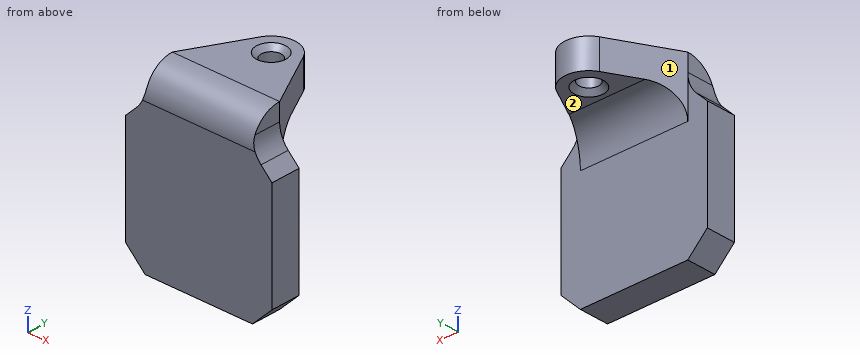
```python
from build123d import *

# Parameters (mm, degrees)
SKETCH_1_W      = 30
SKETCH_1_H      = 30
EXTRUDE_1_DEPTH = 6
CHAMFER_1_SIZE  = 4
SKETCH_2_R      = 2
EXTRUDE_2_DEPTH = 6
FILLET_1_R      = 6
FILLET_2_R      = 6
FILLET_3_R      = 6
CHAMFER_2_SIZE  = 1


with BuildPart() as part:
    # 草图1 → 凸台-拉伸1 (new body)
    with BuildSketch(Plane(origin=(0, 0, 0), x_dir=(1, 0, 0), z_dir=(0, 1, 0))):
        Rectangle(SKETCH_1_W, SKETCH_1_H)
    extrude(amount=EXTRUDE_1_DEPTH)

    # 倒角1
    chamfer_1_edges = [part.edges().sort_by_distance(p)[0] for p in [
        (15, 3, 15),
        (-15, 3, 15),
        (-15, 3, -15),
        (15, 3, -15),
    ]]
    chamfer(chamfer_1_edges, length=CHAMFER_1_SIZE)

    # 草图2 → 凸台-拉伸2 (add)
    with BuildSketch(Plane.XY.offset(15)):
        with BuildLine():
            Line((-11, 6), (-4.411764706, 18.352941176))
            ThreePointArc((-4.411764706, 18.352941176), (0, 21), (4.411764706, 18.352941176))
            Line((4.411764706, 18.352941176), (11, 6))
            Line((11, 6), (11, 0))
            Line((11, 0), (-11, 0))
            Line((-11, 0), (-11, 6))
        make_face()
        with Locations((0, 16)):
            Circle(SKETCH_2_R, mode=Mode.SUBTRACT)
    extrude(amount=EXTRUDE_2_DEPTH)

    # 圆角1
    fillet_1_edges = [part.edges().sort_by_distance(p)[0] for p in [
        (0, 0, 21),
    ]]
    fillet(fillet_1_edges, radius=FILLET_1_R)

    # 圆角2
    # the kernel refuses this fillet: 6 mm, written as the material it adds along each edge
    with BuildSketch(Plane(origin=(-11, 0, 15), x_dir=(-0.7071067811865481, 0, -0.7071067811865467), z_dir=(0, 1, 0))) as fillet_2_piece_1_section:
        with BuildLine():
            CenterArc((FILLET_2_R * 0.414213562373, FILLET_2_R), FILLET_2_R, 225, 45)
            Line((-FILLET_2_R * 0.292893218813, FILLET_2_R * 0.292893218813), (0, 0))
            Line((0, 0), (FILLET_2_R * 0.414213562373, 0))
        make_face()
    fillet_2_piece_1 = extrude(amount=6, mode=Mode.PRIVATE)
    fillet_2_piece_1 = split(fillet_2_piece_1, bisect_by=Plane(origin=(-11.980240057, 0.038623377, 15), z_dir=(0, 0, -1)), keep=Keep.TOP, mode=Mode.PRIVATE)
    add(fillet_2_piece_1)
    with BuildSketch(Plane(origin=(-11, -6.213203436, 15), x_dir=(-0.7071067811865482, 0, -0.7071067811865468), z_dir=(0, 1, 0))) as fillet_2_piece_2_section:
        with BuildLine():
            CenterArc((FILLET_2_R * 0.414213562373, FILLET_2_R), FILLET_2_R, 225, 45)
            Line((-FILLET_2_R * 0.292893218813, FILLET_2_R * 0.292893218813), (0, 0))
            Line((0, 0), (FILLET_2_R * 0.414213562373, 0))
        make_face()
    fillet_2_piece_2 = extrude(amount=12.213203436, mode=Mode.PRIVATE)
    fillet_2_piece_2 = fillet_2_piece_2 & Plane(origin=(-11.156065336, 6, 15), x_dir=(0, -1, 0), z_dir=(-1, 0, 0)) * Cylinder(6, 35, mode=Mode.PRIVATE)
    add(fillet_2_piece_2)
    with BuildSketch(Plane(origin=(11, 0, 15), x_dir=(0.7071067811865482, 0, -0.7071067811865468), z_dir=(0, 1, 0))) as fillet_2_piece_3_section:
        with BuildLine():
            CenterArc((FILLET_2_R * 0.414213562373, -FILLET_2_R), FILLET_2_R, 90, 45)
            Line((-FILLET_2_R * 0.292893218813, -FILLET_2_R * 0.292893218813), (0, 0))
            Line((0, 0), (FILLET_2_R * 0.414213562373, 0))
        make_face()
    fillet_2_piece_3 = extrude(amount=6, mode=Mode.PRIVATE)
    fillet_2_piece_3 = split(fillet_2_piece_3, bisect_by=Plane(origin=(11.980240057, 0.038623377, 15), z_dir=(0, 0, -1)), keep=Keep.TOP, mode=Mode.PRIVATE)
    add(fillet_2_piece_3)
    with BuildSketch(Plane(origin=(11, -6.213203436, 15), x_dir=(0.7071067811865476, 0, -0.7071067811865476), z_dir=(0, 1, 0))) as fillet_2_piece_4_section:
        with BuildLine():
            CenterArc((FILLET_2_R * 0.414213562373, -FILLET_2_R), FILLET_2_R, 90, 45)
            Line((-FILLET_2_R * 0.292893218813, -FILLET_2_R * 0.292893218813), (0, 0))
            Line((0, 0), (FILLET_2_R * 0.414213562373, 0))
        make_face()
    fillet_2_piece_4 = extrude(amount=12.213203436, mode=Mode.PRIVATE)
    fillet_2_piece_4 = fillet_2_piece_4 & Plane(origin=(11.156065336, 6, 15), x_dir=(0, -1, 0), z_dir=(-1, 0, 0)) * Cylinder(6, 35, mode=Mode.PRIVATE)
    add(fillet_2_piece_4)

    # 圆角3
    fillet_3_edges = [part.edges().sort_by_distance(p)[0] for p in [
        (0, 6, 15),
    ]]
    fillet(fillet_3_edges, radius=FILLET_3_R)

    # 倒角2
    chamfer_2_edges = [part.edges().sort_by_distance(p)[0] for p in [
        (-2, 16, 15),
        (-2, 16, 21),
    ]]
    chamfer(chamfer_2_edges, length=CHAMFER_2_SIZE)


solid = part.part
```
Could you check a few things on this model? Use its own coordinates, in mm. Face numbers are marked on the shaded views. A direction names the side the tool comes from. Give positions to 0.01 mm unless a question says otherwise; leave off trailing zeros. Order: outer loops, then holes, each group sorted by start corner. A loop starts at its lowest first (then second) coordinate and runs counter-clockwise, first axis right, second up.
Q1. I'm going to push flat-ended pins straight in: P1, Ø9, axis at x = -6, z = 2.5, coming from the +Y side; P2, Ø4.5, axis at x = -2, y = 17, coming from the -Z side; P3, Ø4, axis at y = 6, z = 17.5, coming from the +X side. Where does each tip first touch, or does it pass through?
Q2. If I drill on line 1 along Y through (x, z) = (-12.5, -3.5); line 2 along Y through (x, z) = (0, 19.1); line 3 along Z through (x, y) = (-0.5, 13), over which ranges is the centre line in solid material (lowest first)?
Q3. Suppose I cut it at D-D, the plane z = 10. Write out the boundary of the cut face in (x, y), and give its area (3 significant figures).
Q4. Suppose I cut it at B-B, the plane y = 16. Write out the boundary of the cut face in (x, z), and give its area (3 significant figures).
Q5. For the marked faces 1 and 2, which set-ups out of +Z, -Z, +X, -X, +Y, -Y let a thin tool reach every point of the face, with its end or its side?
Q6. Suppose I cut it at C-C, the plane z = 19.5. Write out the boundary of the cut face in (x, y), and give its area (3 significant figures).
Q7. Suppose I cut it at A-A, the plane x = 0. Write out the boundary of the cut face in (y, z).
Solution:
1. P1: stops at y = 6
1. P2: stops at z = 15
1. P3: stops at x = 11.34
2. line 1: y = 0 to 6
2. line 2: y = 1.62 to 14, 18 to 21
2. line 3: z = 15 to 21
3. outline: (-15, 0) - (15, 0) - (15, 6) - (11, 6) - (10.96, 6.08) - (-10.96, 6.08) - (-11, 6) - (-15, 6) - close
3. area: 182 mm2
4. outline: (-5.67, 15) - (-3, 15) - (-2, 16) - (-2, 20) - (-3, 21) - (-5.67, 21) - close; (2, 16) - (3, 15) - (5.67, 15) - (5.67, 21) - (3, 21) - (2, 20) - close
4. area: 42.0 mm2
5. face 1: +Z, -Z, -X, +Y
5. face 2: -Z, +X, -X, +Y
6. outline: (-11, 2.03) - (11, 2.03) - (11, 6) - (4.41, 18.35) arc R5 ccw to (-4.41, 18.35) - (-11, 6) - close; hole circle Ø4 at (0, 16)
6. area: 282 mm2
7. outline: (0, -15) - (6, -15) - (6, 9) arc R6 cw to (12, 15) - (13, 15) - (14, 16) - (14, 20) - (13, 21) - (6, 21) arc R6 ccw to (0, 15) - close; (18, 16) - (19, 15) - (21, 15) - (21, 21) - (19, 21) - (18, 20) - close
